For this review, take the finished solid that the model builds, in its own axes (mm). Face numbers are marked on the shaded views. A direction names the side the tool comes from. Give positions to 0.01 mm unless a question says otherwise; leave off trailing zeros. Order: outer loops, then holes, each group sorted by start corner. A loop starts at its lowest first (then second) coordinate and runs counter-clockwise, first axis right, second up. Notation, with made-up numbers: (51.25, -16) -> (103.25, -16) arc R16 cw to (103.25, 3) -> close; hole circle Ø8 at (81, 58). An arc over 180 degrees is marked (long way). Return JSON: item names as keys, results as strings. Group by question number.
1) For the marked faces 1, 2 and 3, list the 3-axis set-ups (+Z, -Z, +X, -X, +Y, -Y) from which the entire face can be reached by the end or side of a thin tool; tool diameter is ignored.
2) The part is to be moulded in two halves that separate along Z. For the marked faces 4, 5 and 6, say which applies: released by +Z, released by -Z, zero draft, split by the parting line, or undercut.
3) Add section C-C (y = 59). Give the boundary of the cut face in (x, z), then the cut area to 3 significant figures.
4) Add section A-A (x = -39). Give the boundary of the cut face in (y, z).
5) Add section D-D (x = 25). Give the boundary of the cut face in (y, z), then the cut area to 3 significant figures.
6) To check wall thickness, follow line 1 along X through (y, z) = (49.5, -14.5); line 2 along X through (y, z) = (17.5, -25); line 3 along X through (y, z) = (34, 41). State the ranges of each line that lie inside material, in increasing order.
7) Add section B-B (z = -28.5). Give the boundary of the cut face in (x, y).
8) Insertion check: P1, Ø3, axis at y = 27, z = 47.5, coming from the +X side; P2, Ø3, axis at y = 6.5, z = -1, coming from the +X side; P3, Ø1.5, axis at x = 47, y = 11.5, coming from the +Z side. Each pin has a flat end and moves straight along its axis. Give the tip position at first contact, or say it passes through.
from build123d import *

# Parameters (mm, degrees)
F1_DEPTH = 63.5


with BuildPart() as f1:
    # F0 (on Front) → F1 (new body)
    with BuildSketch(Plane.XZ):
        Polygon((0, 86.047202), (-22.497155, 49.544945), (-74.853934, 47.332685), (-33.558447, 11.199133), (-33.401991, 11.005372), (-44.619739, -38.207963), (0.404536, -12.584389), (55.13744, -37.764196), (36.865104, 11.936555), (75.948335, 47.332685), (23.222847, 50.651066), align=None)
    extrude(amount=-F1_DEPTH)


solid = f1.part
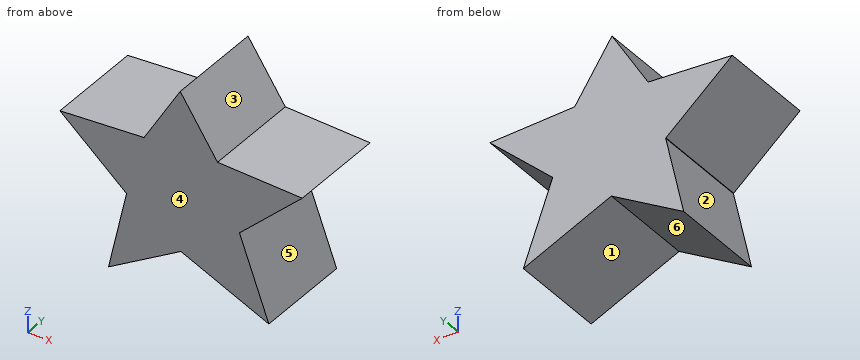
Evaluation:
{
 "1": {"face 1": "-Z, +Y, -Y", "face 2": "-X, +Y, -Y", "face 3": "+Z, +X, +Y, -Y"},
 "2": {"face 4": "zero draft", "face 5": "undercut", "face 6": "released by -Z"},
 "3": {"outline": "(-74.85, 47.33) -> (-33.56, 11.2) -> (-33.4, 11.01) -> (-44.62, -38.21) -> (0.4, -12.58) -> (55.14, -37.76) -> (36.87, 11.94) -> (75.95, 47.33) -> (23.22, 50.65) -> (0, 86.05) -> (-22.5, 49.54) -> close", "area": "8,000 mm^2"},
 "4": {"outline": "(0, -35.01) -> (63.5, -35.01) -> (63.5, -13.55) -> (0, -13.55) -> close; (0, 15.96) -> (63.5, 15.96) -> (63.5, 48.85) -> (0, 48.85) -> close"},
 "5": {"outline": "(0, -23.9) -> (63.5, -23.9) -> (63.5, 50.54) -> (0, 50.54) -> close", "area": "4,730 mm^2"},
 "6": {"line 1": "-39.22 to -2.96, 4.57 to 46.58", "line 2": "-41.61 to -21.41, 27.39 to 50.44", "line 3": "-67.62 to 68.96"},
 "7": {"outline": "(-42.41, 0) -> (-27.56, 0) -> (-27.56, 63.5) -> (-42.41, 63.5) -> close; (35, 0) -> (51.73, 0) -> (51.73, 63.5) -> (35, 63.5) -> close"},
 "8": {"P1": "x = 75.95", "P2": "x = 42.17", "P3": "z = 49.2"}
}
